Verification items for the finished model (mm, model axes). Face numbers are marked on the shaded views. A direction names the side the tool comes from. Coordinates: 2 decimals unless noted, no trailing zeros. Loops run counter-clockwise (first coordinate to the right, second up) from the corner with the lowest first, then second, coordinate; pieces in that order, holes last. Notation, with made-up numbers: (81, 48.5) - (124, 48.5) arc R13 cw to (124, 70.5) - close; hole circle Ø2 at (20, -7.5). An arc over 180 degrees is marked (long way). One line per item, written item: value. Start each with the question number.
(1) Section check A-A (x = 0). Record the boundary of the cut face in (y, z).
(2) Section check C-C (z = 43). Record the boundary of the cut face in (x, y), plus the area to 3 significant figures.
(3) Set-up check for the marked faces 1 and 2: record each of +Z, -Z, +X, -X, +Y, -Y from which the full face is reachable in a straight line by a thin tool's end or side.
(4) Thickness scan on probe 1 along Z at (x, y) = (-4, -12.5); probe 2 along Z at (x, y) = (-4, 4); probe 3 along X at (y, z) = (0.75, -20). Record the ranges inside material, lowest first. Write a range as [from, to].
(5) Section check D-D (z = 13). Record the boundary of the cut face in (x, y), plus the area to 3 significant figures.
(6) Gauge pin test, flat ends, axial feed: P1, Ø1.5, axis at x = -9.5, z = -11.5, coming from the -Y side; P2, Ø3, axis at y = -10.5, z = -5, coming from the +X side; P3, Ø1.5, axis at x = 8, z = 33, coming from the -Y side. Record the tip position at first contact, or that the pin passes through.
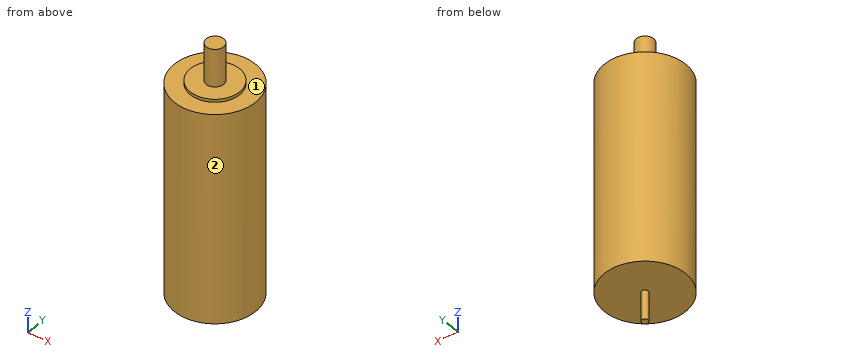
```python
from build123d import *

# Parameters (mm, degrees)
SKETCH1_R           = 14
BOSS_EXTRUDE1_DEPTH = 36.2
SKETCH2_R           = 8.5
BOSS_EXTRUDE2_DEPTH = 1
SKETCH3_R           = 3
BOSS_EXTRUDE3_DEPTH = 13
SKETCH5_R           = 1.15
BOSS_EXTRUDE4_DEPTH = 10


with BuildPart() as part:
    # Sketch1 → Boss-Extrude1 (new, symmetric)
    with BuildSketch(Plane.XY):
        with Locations(Location((0, 0, 0), (0, 0, 180))):
            Circle(SKETCH1_R)
    extrude(amount=BOSS_EXTRUDE1_DEPTH, both=True)

    # Sketch2 → Boss-Extrude2 (add, symmetric)
    with BuildSketch(Plane.XY.offset(36.2)):
        Circle(SKETCH2_R)
    extrude(amount=BOSS_EXTRUDE2_DEPTH, both=True)

    # Sketch3 → Boss-Extrude3 (add)
    with BuildSketch(Plane.XY.offset(37.2)):
        with Locations(Location((0, 0, 0), (0, 0, 180))):
            Circle(SKETCH3_R)
    extrude(amount=BOSS_EXTRUDE3_DEPTH)

    # Sketch5 → Boss-Extrude4 (add)
    with BuildSketch(Plane(origin=(0, 0, -36.2), x_dir=(-1, 0, 0), z_dir=(0, 0, -1))):
        with Locations(Location((0, 0, 0), (0, 0, 180))):
            Circle(SKETCH5_R)
    extrude(amount=BOSS_EXTRUDE4_DEPTH)


solid = part.part
```
Responses:
1. outline: (-14, -36.2) - (-1.15, -36.2) - (-1.15, -46.2) - (1.15, -46.2) - (1.15, -36.2) - (14, -36.2) - (14, 36.2) - (8.5, 36.2) - (8.5, 37.2) - (3, 37.2) - (3, 50.2) - (-3, 50.2) - (-3, 37.2) - (-8.5, 37.2) - (-8.5, 36.2) - (-14, 36.2) - close
2. outline: circle Ø6 at (0, 0)
2. area: 28.3 mm²
3. face 1: +Z
3. face 2: +Z, -Z
4. probe 1: z = [-36.2, 36.2]
4. probe 2: z = [-36.2, 37.2]
4. probe 3: x = [-13.98, 13.98]
5. outline: circle Ø28 at (0, 0)
5. area: 616 mm²
6. P1: stops at y = -10.93
6. P2: stops at x = 10.72
6. P3: stops at y = -11.98
